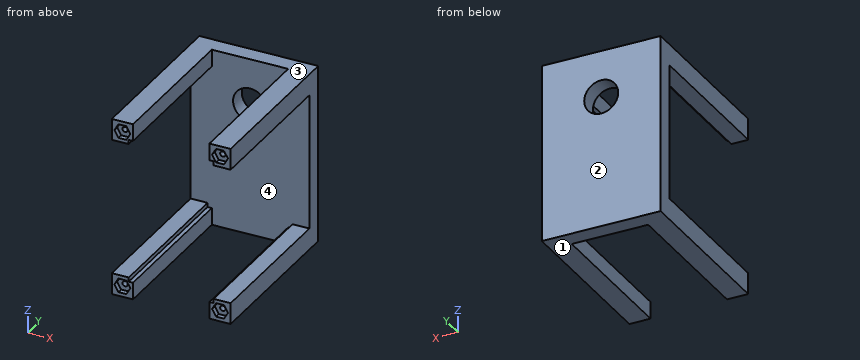
```python
from build123d import *

# Parameters (mm, degrees)
SKETCH1_W               = 71.12
SKETCH1_H               = 106.68
BOSS_EXTRUDE1_DEPTH     = 101.6
SHELL1_T                = -10.16
SKETCH3_R               = 1.5875
CUT_EXTRUDE1_DEPTH      = 10.16
SKETCH4_W               = 81.28
SKETCH4_H               = 91.44
CUT_EXTRUDE2_DEPTH      = 72.12
CUT_EXTRUDE3_DEPTH      = 3.175
SKETCH7_W               = 45.72
SKETCH7_H               = 91.44
CUT_EXTRUDE4_DEPTH      = 1
CUT_EXTRUDE4_DEPTH_BACK = 107.68
CUT_EXTRUDE5_REACH      = 103.6
SKETCH8_R               = 10.16


with BuildPart() as part:
    # Sketch1 → Boss-Extrude1 (new body)
    with BuildSketch(Plane(origin=(0, 0, 0), x_dir=(1, 0, 0), z_dir=(0, 1, 0))):
        with Locations((35.56, 53.34)):
            Rectangle(SKETCH1_W, SKETCH1_H)
    extrude(amount=BOSS_EXTRUDE1_DEPTH)

    # Shell1
    shell1_openings = [part.faces().sort_by_distance(p)[0] for p in [
        (35.56, 0, -53.34),
    ]]
    offset(amount=SHELL1_T, openings=shell1_openings, kind=Kind.INTERSECTION)

    # Sketch3 → Cut-Extrude1 (cut)
    with BuildSketch(Plane.XZ):
        with Locations((6.35, -6.35)):
            Circle(SKETCH3_R)
        with Locations((64.77, -6.35)):
            Circle(SKETCH3_R)
        with Locations((64.77, -100.33)):
            Circle(SKETCH3_R)
        with Locations((6.35, -100.33)):
            Circle(SKETCH3_R)
    extrude(amount=-CUT_EXTRUDE1_DEPTH, mode=Mode.SUBTRACT)

    # Sketch4 → Cut-Extrude2 (cut, through all)
    with BuildSketch(Plane.ZY):
        with Locations((-53.34, 45.72)):
            Rectangle(SKETCH4_W, SKETCH4_H)
    extrude(amount=-CUT_EXTRUDE2_DEPTH, mode=Mode.SUBTRACT)

    # Sketch6 → Cut-Extrude3 (cut)
    with BuildSketch(Plane.XZ):
        Polygon((69.536026472, -6.35), (67.153013236, -2.2225), (62.386986764, -2.2225), (60.003973528, -6.35), (62.386986764, -10.4775), (67.153013236, -10.4775), align=None)
        Polygon((11.116026472, -6.35), (8.733013236, -2.2225), (3.966986764, -2.2225), (1.583973528, -6.35), (3.966986764, -10.4775), (8.733013236, -10.4775), align=None)
        Polygon((69.536026472, -100.33), (67.153013236, -96.2025), (62.386986764, -96.2025), (60.003973528, -100.33), (62.386986764, -104.4575), (67.153013236, -104.4575), align=None)
        Polygon((11.116026472, -100.33), (8.733013236, -96.2025), (3.966986764, -96.2025), (1.583973528, -100.33), (3.966986764, -104.4575), (8.733013236, -104.4575), align=None)
    extrude(amount=-CUT_EXTRUDE3_DEPTH, mode=Mode.SUBTRACT)

    # Sketch7 → Cut-Extrude4 (cut, two sides)
    with BuildSketch(Plane(origin=(0, 0, -106.68), x_dir=(-1, 0, 0), z_dir=(0, 0, -1))) as cut_extrude4_sk:
        with Locations((-35.56, 45.72)):
            Rectangle(SKETCH7_W, SKETCH7_H)
    extrude(amount=CUT_EXTRUDE4_DEPTH, mode=Mode.SUBTRACT)
    extrude(cut_extrude4_sk.sketch, amount=-CUT_EXTRUDE4_DEPTH_BACK, mode=Mode.SUBTRACT)

    # Sketch8 → Cut-Extrude5 (cut, up to next)
    with BuildSketch(Plane(origin=(0, 101.6, 0), x_dir=(1, 0, 0), z_dir=(0, 1, 0)), mode=Mode.PRIVATE) as cut_extrude5_sk1:
        with Locations((35.56, 27.94)):
            Circle(SKETCH8_R)
    cut_extrude5_tool1 = extrude(cut_extrude5_sk1.sketch, amount=-CUT_EXTRUDE5_REACH, mode=Mode.PRIVATE) & part.part
    add(cut_extrude5_tool1.solids().sort_by_distance((35.56, 101.6, -27.94))[0], mode=Mode.SUBTRACT)


solid = part.part
```
Verification items for the finished model (mm, model axes). Face numbers are marked on the shaded views. Coordinates: 2 decimals unless noted, no trailing zeros. Loops run counter-clockwise (first coordinate to the right, second up) from the corner with the lowest first, then second, coordinate; pieces in that order, holes last. Notation, with made-up numbers: (83.5, 4.25) -> (110.5, 4.25) arc R6 cw to (110.5, 13.25) -> close; hole circle Ø10 at (40, 85). An arc over 180 degrees is marked (long way). Answer in a Markdown table with one row per item. Add a question column.
1. Depth check by flat-ended pin: P1, Ø4, axis at x = 65.5, z = -101, coming from the -Y side (3 decimals). Enter the tip coordinate at first touch or a pass-through.
2. Section check D-D, the plane z = -86. Enter the section's corners in (x, y).
3. Section check A-A, the plane y = 75.5. Enter the section's corners in (x, z), then the cut area to 3 significant figures.
4. Section check C-C, the plane x = 64.77. Enter the section's corners in (y, z) (1 decimal).
5. Draft check along Z on the marked faces 1, 2, 3 and 4. Enter one of: +Z half, -Z half, draft (parallel to the pull), parting line (faces both ways), or undercut.
6. Material ranges on probe 1 along Z at (x, y) = (64.77, 6.75); probe 2 along X at (y, z) = (6.75, -100.33); probe 3 along Z at (x, y) = (59, 86.5), recorded low to high. Write a range as [from, to].
7. Section check B-B, the plane x = 31. Enter the section's corners in (y, z).
Derived:
| question | item | result |
|---|---|---|
| 1 | P1 | stops at y = 3.175 |
| 2 | outline | (0, 91.44) -> (71.12, 91.44) -> (71.12, 101.6) -> (0, 101.6) -> close |
| 3 | outline | (0, -106.68) -> (12.7, -106.68) -> (12.7, -96.52) -> (10.16, -96.52) -> (10.16, -93.98) -> (0, -93.98) -> close; (0, -12.7) -> (10.16, -12.7) -> (10.16, -10.16) -> (12.7, -10.16) -> (12.7, 0) -> (0, 0) -> close; (58.42, -106.68) -> (71.12, -106.68) -> (71.12, -93.98) -> (60.96, -93.98) -> (60.96, -96.52) -> (58.42, -96.52) -> close; (58.42, -10.16) -> (60.96, -10.16) -> (60.96, -12.7) -> (71.12, -12.7) -> (71.12, 0) -> (58.42, 0) -> close |
| 3 | area | 619 mm² |
| 4 | outline | (0, -106.7) -> (101.6, -106.7) -> (101.6, 0) -> (0, 0) -> (0, -2.2) -> (3.2, -2.2) -> (3.2, -4.8) -> (10.2, -4.8) -> (10.2, -7.9) -> (3.2, -7.9) -> (3.2, -10.5) -> (0, -10.5) -> (0, -12.7) -> (91.4, -12.7) -> (91.4, -94) -> (0, -94) -> (0, -96.2) -> (3.2, -96.2) -> (3.2, -98.7) -> (10.2, -98.7) -> (10.2, -101.9) -> (3.2, -101.9) -> (3.2, -104.5) -> (0, -104.5) -> close |
| 5 | face 1 | -Z half |
| 5 | face 2 | draft |
| 5 | face 3 | +Z half |
| 5 | face 4 | undercut |
| 6 | probe 1 | z = [-106.68, -101.92], [-98.74, -93.98], [-12.7, -7.94], [-4.76, 0] |
| 6 | probe 2 | x = [0, 4.76], [7.94, 12.7], [58.42, 63.18], [66.36, 71.12] |
| 6 | probe 3 | z = [-106.68, -96.52], [-10.16, 0] |
| 7 | outline | (91.44, -106.68) -> (101.6, -106.68) -> (101.6, -37.02) -> (91.44, -37.02) -> close; (91.44, -18.86) -> (101.6, -18.86) -> (101.6, 0) -> (91.44, 0) -> close |
